Check sheet for the modelled part. Datum: model origin and axes. Units: mm. A direction names the side the tool comes from. Round coordinates to 2 decimals unless told otherwise and drop trailing zeros. Order: outer loops, then holes, each group sorted by start corner. A loop starts at its lowest first (then second) coordinate and runs counter-clockwise, first axis right, second up.
Autodesk Inventor part; units mm, degrees
ref_plane "YZ Plane" through (0, 0, 0) normal (1, 0, 0) x (0, 1, 0)
ref_plane "XZ Plane" through (0, 0, 0) normal (0, 1, 0) x (-1, 0, 0)
ref_plane "XY Plane" through (0, 0, 0) normal (0, 0, 1) x (1, 0, 0)
sketch "Sketch1" plane through (0, 0, 0) normal (0, 1, 0) x (-1, 0, 0)
  line L0 (0, 0) -> (680, 0)
  line L1 (680, 0) -> (680, -1118)
  line L2 (680, -1118) -> (0, -1118)
  line L3 (0, -1118) -> (0, 0)
  dimension "d0" = 680
  dimension "d1" = 1118
extrude "Extrusion1" add sketch "Sketch1" along normal blind 50
sketch "Sketch2" plane through (0, 50, 0) normal (0, 1, 0) x (1, 0, 0)
  line L0 (-50, 50) -> (-630, 50)
  line L1 (-630, 50) -> (-630, 1068)
  line L2 (-630, 1068) -> (-50, 1068)
  line L3 (-50, 1068) -> (-50, 50)
  point P0 (0, 0)
  dimension "d4" = 580
  dimension "d5" = 1018
extrude "Extrusion2" cut sketch "Sketch2" against normal blind 50
sketch "Sketch3" plane through (0, 50, 0) normal (0, 1, 0) x (1, 0, 0)
  point P0 (0, 0)
sketch "Sketch4" plane through (0, 50, 0) normal (0, 1, 0) x (1, 0, 0)
  line L0 (-680, 0) -> (0, 0)
  line L1 (-251, 0) -> (-429, 0)
  line L2 (-429, 0) -> (-429, 50)
  line L3 (-429, 50) -> (-251, 50)
  line L4 (-251, 50) -> (-251, 0)
  dimension "d8" = 178
  dimension "d9" = 50
extrude "Extrusion3" add sketch "Sketch4" along normal blind 254
sketch "Sketch5" plane through (0, 50, 0) normal (0, 1, 0) x (1, 0, 0)
  line L0 (0, 1118) -> (-680, 1118)
  line L1 (-630, 1068) -> (-50, 1068)
  line L2 (-251, 1118) -> (-429, 1118)
  line L3 (-429, 1118) -> (-429, 1068)
  line L4 (-429, 1068) -> (-251, 1068)
  line L5 (-251, 1068) -> (-251, 1118)
  point P0 (0, 0)
  dimension "d12" = 178
extrude "Extrusion4" add sketch "Sketch5" along normal blind 254
sketch "Sketch6" plane through (0, 304, 0) normal (0, 1, 0) x (1, 0, 0)
  circle A0 centre (-340, 25) radius 25
  point P0 (0, 0)
  dimension "d15" = 50
extrude "Extrusion5" add sketch "Sketch6" along normal blind 450
sketch "Sketch7" plane through (0, 304, 0) normal (0, 1, 0) x (1, 0, 0)
  circle A0 centre (-340, 1093) radius 25
  point P0 (0, 0)
  dimension "d18" = 50
extrude "Extrusion6" add sketch "Sketch7" along normal blind 450
sketch "Sketch8" plane through (-340, 754, -25) normal (0, 1, 0) x (1, 0, 0)
  line L0 (-340, -25) -> (340, -25)
  line L1 (25, -25) -> (-25, -25)
  line L2 (-25, -25) -> (-25, 1093)
  line L3 (-25, 1093) -> (25, 1093)
  line L4 (25, 1093) -> (25, -25)
  dimension "d21" = 50
  dimension "d22" = 1118
extrude "Extrusion7" add sketch "Sketch8" along normal blind 50
sketch "Sketch9" plane through (-315, 754, -25) normal (1, 0, 0) x (0, 0, -1)
  line L0 (0, 0) -> (-25, 0)
  line L1 (-25, 0) -> (25, 0)
  line L2 (25, 0) -> (25, 50)
  line L3 (25, 50) -> (-25, 50)
  line L4 (-25, 50) -> (-25, 0)
  point P0 (-25, -754)
  dimension "d25" = 50
  dimension "d26" = 50
extrude "Extrusion8" add sketch "Sketch9" along normal blind 315
sketch "Sketch10" plane through (-315, 754, -1093) normal (1, 0, 0) x (0, 0, -1)
  line L0 (25, 0) -> (25, 50)
  line L1 (25, 0) -> (-25, 0)
  line L2 (-25, 0) -> (-25, 50)
  line L3 (-25, 50) -> (25, 50)
  line L4 (25, 50) -> (25, 0)
  point P0 (-1093, -754)
  dimension "d29" = 50
  dimension "d30" = 50
extrude "Extrusion9" add sketch "Sketch10" along normal blind 315
sketch "Sketch11" plane through (-365, 754, -1093) normal (-1, 0, 0) x (0, 0, 1)
  line L0 (-25, 50) -> (1093, 50)
  line L1 (-25, 50) -> (25, 50)
  line L2 (25, 50) -> (25, 0)
  line L3 (25, 0) -> (-25, 0)
  line L4 (-25, 0) -> (-25, 50)
  point P0 (1093, -754)
  dimension "d33" = 50
  dimension "d34" = 50
extrude "Extrusion10" add sketch "Sketch11" along normal blind 315
sketch "Sketch12" plane through (-365, 754, -25) normal (-1, 0, 0) x (0, 0, 1)
  line L0 (-1043, 50) -> (25, 50)
  line L1 (25, 50) -> (-25, 50)
  line L2 (-25, 50) -> (-25, 0)
  line L3 (-25, 0) -> (25, 0)
  line L4 (25, 0) -> (25, 50)
  point P0 (25, -754)
  dimension "d37" = 50
  dimension "d38" = 50
extrude "Extrusion11" add sketch "Sketch12" along normal blind 315
sketch "Sketch13" plane through (0, 754, -1118) normal (0, 0, -1) x (-1, 0, 0)
  line L0 (680, 0) -> (680, 50)
  line L1 (680, 50) -> (610, 50)
  line L2 (610, 50) -> (610, 80.718)
  line L3 (650, 150) -> (680, 150)
  line L4 (680, 150) -> (680, 50)
  line L5 (0, 50) -> (70, 50)
  line L6 (70, 50) -> (70, 80.718)
  line L7 (30, 150) -> (0, 150)
  line L8 (0, 150) -> (0, 50)
  line L9 (650, 150) -> (610, 80.718)
  line L10 (650, 150) -> (680, 150) construction
  line L11 (30, 150) -> (70, 80.718)
  point P0 (0, -754)
extrude "Extrusion12" add sketch "Sketch13" against normal blind 1118
sketch "Sketch14" plane through (0, 754, -25) normal (1, 0, 0) x (0, 0, -1)
  line L0 (25, 50) -> (1043, 50)
  line L1 (1043, 50) -> (25, 50)
  line L2 (25, 50) -> (25, 150)
  line L3 (25, 150) -> (1043, 150)
  line L4 (1043, 150) -> (1043, 50)
  point P0 (-25, -754)
extrude "Extrusion13" cut sketch "Sketch14" against normal blind 1118
sketch "Sketch15" plane through (-340, 754, 0) normal (0, 0, 1) x (1, 0, 0)
  circle A0 centre (325, 140) radius 50
  circle A1 centre (-325, 140) radius 50
  line L0 (340, 0) -> (340, 150)
  line L1 (340, 0) -> (340, 150)
  line L2 (0, 0) -> (-340, 0)
  line L3 (0, 0) -> (340, 0)
  line L4 (340, 0) -> (340, 150)
  line L5 (340, 150) -> (310, 150)
  line L6 (310, 150) -> (270, 80.718)
  line L7 (270, 80.718) -> (270, 50)
  line L8 (270, 50) -> (-270, 50)
  line L9 (-270, 50) -> (-270, 80.718)
  line L10 (-270, 80.718) -> (-310, 150)
  line L11 (-310, 150) -> (-340, 150)
  line L12 (-340, 0) -> (-340, 150)
  point P0 (340, -754)
  point P1 (340, 92.303)
  point P2 (286.0942, 108.594)
extrude "Extrusion14" add sketch "Sketch15" against normal blind 1118 contours A0 L0 L5 L6 | L12 L11 L10 A1 | A1 L10 L11 L12 picked at (325.7082, 163.3183)
move or copy body "Rotate1" bodies to move or copy 1 copy no rotation origin (0, 0, 0) rotation axis (1, 0, 0) rotation angle 180 translate (0, 1788, -1118)
sketch "Sketch16" plane through (0, 1034, 0) normal (1, 0, 0) x (0, 0, -1)
  line L0 (50, 0) -> (50, -92.303)
  line L1 (50, -72.2577) -> (1068, -72.2577)
  line L2 (1068, -72.2577) -> (1068, -234.0796)
  line L3 (1068, -234.0796) -> (50, -234.0796)
  line L4 (50, -234.0796) -> (50, -72.2577)
  point P0 (0, -1034)
  dimension "d58" = 1018
extrude "Extrusion15" cut sketch "Sketch16" against normal blind 1118
sketch "Sketch17" plane through (-680, 1034, -1118) normal (-1, 0, 0) x (0, 0, 1)
  line L0 (1118, -80.718) -> (1068, -80.718)
  line L1 (1068, -80.718) -> (50, -80.718)
  line L2 (50, -80.718) -> (50, -329.635)
  line L3 (50, -329.635) -> (1068, -329.635)
  line L4 (1068, -329.635) -> (1068, -80.718)
  point P0 (1118, -1034)
  dimension "d61" = 1018
extrude "Extrusion16" cut sketch "Sketch17" against normal blind 1118
properties part number "Human-Subject-Cart"
Item 1: Access from +Z, -Z, +X, -X, +Y, -Y to the whole of each face (thin tool, end or side, straight path). Record for faces 1 (the flat face through (-610, 969, -1093)), 2 (the flat face through (0, 987, -25)), 3 (the flat face through (-630, 1763, -566)).
Answer:
face 1: +Z, -Z, -Y
face 2: +Z, -Z, +X, +Y
face 3: +Y, -Y
Item 2: Sectioned sample at C-C (x = -588.5). Record the cut outline in (y, z), and give its area (3 significant figures).
Answer:
outline: (984, -1118) - (1034, -1118) - (1034, -1068) - (984, -1068) - close; (984, -50) - (1034, -50) - (1034, 0) - (984, 0) - close; (1738, -1118) - (1788, -1118) - (1788, -1068) - (1738, -1068) - close; (1738, -50) - (1788, -50) - (1788, 0) - (1738, 0) - close
area: 10,000 mm2
Item 3: Scan lines: line 1 along Z through (x, y) = (-399.5, 1532); line 2 along Y through (x, z) = (-350.5, -673.5). Record each from-to range of solid material in increasing order.
Answer:
line 1: z = -1118 to -1068, -50 to 0
line 2: y = 984 to 1034
Item 4: Go/stop test with flat-tipped pins: P1, Ø15, axis at y = 1660, z = -23, coming from the +X side; P2, Ø15, axis at y = 1010.5, z = -648.5, coming from the -X side; P3, Ø15.5, axis at y = 967.5, z = -34.5, coming from the +X side. Record where each tip stops, or that it passes through.
Answer:
P1: stops at x = -251
P2: stops at x = -365
P3: stops at x = 0
Item 5: Sectioned sample at D-D (z = -851). Record the cut outline in (x, y), and give its area (3 significant figures).
Answer:
outline: (-680, 1738) - (-630, 1738) - (-630, 1788) - (-680, 1788) - close; (-365, 984) - (-315, 984) - (-315, 1034) - (-365, 1034) - close; (-50, 1738) - (0, 1738) - (0, 1788) - (-50, 1788) - close
area: 7,500 mm2
Item 6: Release check for a two-part mould opening along Z. For faces 4 (the flat face through (-335, 1672, -1118)), 5 (the flat face through (-70, 969, -1093)), 6 (the flat face through (-338, 1034, -556)) record: released by +Z, released by -Z, zero draft, split by the parting line, or undercut.
Answer:
face 4: released by -Z
face 5: zero draft
face 6: undercut
Item 7: Sectioned sample at B-B (y = 894). Record the cut outline in (x, z).
Answer:
outline: (-715, -1118) - (-615, -1118) - (-615, -1068) - (-715, -1068) - close; (-715, -50) - (-615, -50) - (-615, 0) - (-715, 0) - close; (-65, -1118) - (35, -1118) - (35, -1068) - (-65, -1068) - close; (-65, -50) - (35, -50) - (35, 0) - (-65, 0) - close
Item 8: Sectioned sample at A-A (x = -15). Record the cut outline in (y, z).
Answer:
outline: (844, -1118) - (1034, -1118) - (1034, -1068) - (844, -1068) - close; (844, -50) - (1034, -50) - (1034, 0) - (844, 0) - close; (1738, -1118) - (1788, -1118) - (1788, 0) - (1738, 0) - close
